Verification items for the finished model (mm, model axes). A direction names the side the tool comes from. Round coordinates to 2 decimals unless told otherwise and drop trailing zeros. Order: outer loops, then holes, each group sorted by start corner. A loop starts at its lowest first (then second) coordinate and runs counter-clockwise, first axis right, second up. Notation, with made-up numbers: M 59,-27 L 90,-27 A20 ccw 90,-6 Z; hole C 74,72 d7. An arc over 180 degrees is marked long. Return JSON: item names as keys, results as strings. Group by question number.
from build123d import *

# Parameters (mm, degrees)
F0_W      = 61.1153431237
F0_H      = 64.4062012434
F0_W_2    = 55.2647679579
F0_H_2    = 56.5587065648
F1_DEPTH  = 12.7
F2_W      = 55.2647679579
F2_H      = 2.967182314
F3_DEPTH  = 56.896
F5_DEPTH  = 4.318
F6_DEPTH  = 25.4
F7_DEPTH  = 7.874
F8_W      = 3.7420586476
F8_H      = 56.5587065648
F9_DEPTH  = 14.224
F10_DEPTH = 10.922
F11_DEPTH = 6.858


with BuildPart() as f1:
    # F0 (on Top) → F1 (new body)
    with BuildSketch(Plane.XY):
        with Locations((30.5576715618, -32.2031006217)):
            Rectangle(F0_W, F0_H)
        with Locations((30.3483285243, -31.7048091674)):
            Rectangle(F0_W_2, F0_H_2, mode=Mode.SUBTRACT)
    extrude(amount=F1_DEPTH)

    # F2 (on face) → F3 (join)
    with BuildSketch(Plane.XZ.offset(3.425455885)):
        with Locations((30.3483285243, 1.483591157)):
            Rectangle(F2_W, F2_H)
    extrude(amount=F3_DEPTH)

    # F5 (add): a face of the model
    f5_faces = [f1.faces().sort_by_distance(p)[0] for p in [
        (30.5576715618, -0.8878763384, 12.7),
    ]]
    extrude(f5_faces, amount=F5_DEPTH)

    # F4 (on face) → F6 (cut)
    with BuildSketch(Plane.XZ.offset(3.425455885)):
        Polygon((37.590354681, 7.833591157), (37.590354681, 12.7), (30.3483285243, 12.7), (23.1118518859, 12.7), (23.1118518859, 7.833591157), (23.1118518859, 2.967182314), (30.3483285243, 2.967182314), (37.590354681, 2.967182314), align=None)
    extrude(amount=-F6_DEPTH, mode=Mode.SUBTRACT)

    # F7 (cut): a face of the model
    f7_faces = [f1.faces().sort_by_distance(p)[0] for p in [
        (61.1153431237, -32.2031006217, 8.509),
    ]]
    extrude(f7_faces, amount=-F7_DEPTH, mode=Mode.SUBTRACT)

    # F8 (on face) → F9 (join)
    with BuildSketch(Plane.XY.offset(2.967182314)):
        with Locations((51.3703137999, -31.7048091674)):
            Rectangle(F8_W, F8_H)
    extrude(amount=F9_DEPTH)

    # F10 (add): a face of the model
    f10_faces = [f1.faces().sort_by_distance(p)[0] for p in [
        (0, -32.2031006217, 8.509),
    ]]
    extrude(f10_faces, amount=-F10_DEPTH)

    # F11 (cut): a face of the model
    f11_faces = [f1.faces().sort_by_distance(p)[0] for p in [
        (0, -32.2031006217, 8.509),
    ]]
    extrude(f11_faces, amount=-F11_DEPTH, mode=Mode.SUBTRACT)


solid = f1.part
1. Go/stop test with flat-tipped pins: pin 1 (5 mm diameter, centred on x = 34.5, z = 6.5, fed in from +Y); pin 2 (1.5 mm diameter, centred on x = 40.5, y = -54.5, fed in from -Z); pin 3 (23 mm diameter, centred on x = 27.5, y = -32, fed in from +Z). Record where each tip stops, or that it passes through.
2. Cross-section at A-A (x = 25.5). Enter the section's corners in (y, z), plus the area to 3 significant figures.
3. Cross-section at C-C (x = 47.5). Enter the section's corners in (y, z).
4. Cross-section at D-D (y = -28.5). Enter the section's corners in (x, z).
5. Access from +Z, -Z, +X, -X, +Y, -Y to the whole of each face (thin tool, end or side, straight path). Record for faces 1 (the face through (53.241, -33, 8)), 2 (the face through (30, -3.425, 13)), 3 (the face through (30, -2, 12.7)).
6. Cross-section at B-B (z = 14.75). Enter the section's corners in (x, y), plus the area to 3 significant figures.
7. Draft check along Z on faces 4 (the face through (51, -31, 17.191)), 5 (the face through (23.112, -2, 8)), 6 (the face through (49.499, -32, 10)). Enter one of: +Z half, -Z half, draft (parallel to the pull), parting line (faces both ways), or undercut.
8. Thickness scan on line 1 along X through (y, z) = (-58.5, 12); line 2 along Y through (x, z) = (37.5, 15); line 3 along Z through (x, y) = (10.5, -25.5). Record the ranges inside material, lowest first. Write a range as from..to.
Computed:
{
 "1": {"pin 1": "stops at y = -59.98", "pin 2": "stops at z = 0", "pin 3": "stops at z = 2.97"},
 "2": {"outline": "M -64.41,0 L 0,0 L 0,2.97 L -59.98,2.97 L -59.98,17.02 L -64.41,17.02 Z; M -3.43,12.7 L 0,12.7 L 0,17.02 L -3.43,17.02 Z", "area": "268 mm²"},
 "3": {"outline": "M -64.41,0 L 0,0 L 0,17.02 L -3.43,17.02 L -3.43,2.97 L -59.98,2.97 L -59.98,17.02 L -64.41,17.02 Z"},
 "4": {"outline": "M 6.86,0 L 53.24,0 L 53.24,17.19 L 49.5,17.19 L 49.5,2.97 L 10.92,2.97 L 10.92,17.02 L 6.86,17.02 Z"},
 "5": {"face 1": "+Z, -Z, +X, +Y, -Y", "face 2": "+Z", "face 3": "+Y"},
 "6": {"outline": "M 6.86,-64.41 L 53.24,-64.41 L 53.24,0 L 6.86,0 Z; hole M 10.92,-59.98 L 49.5,-59.98 L 49.5,-3.43 L 10.92,-3.43 Z", "area": "805 mm²"},
 "7": {"face 4": "+Z half", "face 5": "undercut", "face 6": "draft"},
 "8": {"line 1": "x = 6.86..10.92, 49.5..53.24", "line 2": "y = -64.41..-59.98, -3.43..0", "line 3": "z = 0..17.02"}
}
